Autodesk Inventor part; units mm, degrees
ref_plane "YZ Plane" through (0, 0, 0) normal (1, 0, 0) x (0, 1, 0)
ref_plane "XZ Plane" through (0, 0, 0) normal (0, 1, 0) x (-1, 0, 0)
ref_plane "XY Plane" through (0, 0, 0) normal (0, 0, 1) x (1, 0, 0)
sketch "Sketch1" plane through (0, 0, 0) normal (0, 1, 0) x (-1, 0, 0)
  line L0 (825, 12.5) -> (-825, 12.5)
  line L1 (-825, 12.5) -> (-825, -12.5)
  line L2 (-825, -12.5) -> (825, -12.5)
  line L3 (825, -12.5) -> (825, 12.5)
  line L4 (825, 12.5) -> (-825, -12.5) construction
  line L5 (-825, 12.5) -> (825, -12.5) construction
  point P0 (0, 0)
  dimension "d0" = 1650
  dimension "d1" = 25
extrude "Plate1" add sketch "Sketch1" along normal blind 3.2
sketch "Sketch2" plane through (825, 0, 9.3) normal (0, 0, 1) x (1, 0, 0)
  line L0 (-1650, 0) -> (0, 0)
  line L1 (0, 0) -> (0, 25)
  line L2 (0, 25) -> (-1650, 25)
  line L3 (-1650, 25) -> (-1650, 0)
edge flange "Flange1" height 25 angle 90 thickness 3.2 bend radius 1.516 thickness toward (0, 0, 1) relief tear relief width 3.2 relief depth 1.6 edges at (0, 3.2, 12.5) wall of the first edge with corners at (-825, 0, 9.3) (825, 0, 9.3) (825, 25, 9.3) (-825, 25, 9.3)
bend "Bend1"
corner "Corner1"
sketch "Sketch3" plane through (825, 25, 9.3) normal (0, 0, -1) x (-1, 0, 0)
  circle A0 centre (105, -10.45) radius 1.5706
  circle A1 centre (285, -10.45) radius 1.5706
  circle A2 centre (465, -10.45) radius 1.5706
  circle A3 centre (825, -10.45) radius 1.5706
  circle A4 centre (1005, -10.45) radius 1.5706
  circle A5 centre (1185, -10.45) radius 1.5706
  circle A6 centre (1365, -10.45) radius 1.5706
  circle A7 centre (1545, -10.45) radius 1.5706
  point P0 (825, -25)
hole "Hole1" at (540, 14.55, 9.3) at (720, 14.55, 9.3) at (360, 14.55, 9.3) at (0, 14.55, 9.3) at (-180, 14.55, 9.3) at (-360, 14.55, 9.3) at (-540, 14.55, 9.3) at (-720, 14.55, 9.3) direction (0, 0, 1) diameter 4.5 depth 3.2 tip angle 118
sketch "Sketch8" plane through (0, 0, 0) normal (0, -1, 0) x (1, 0, 0)
  line L0 (-825, -12.5) -> (825, -12.5)
  line L1 (0, -12.5) -> (0, -2.5)
  line L2 (0, -2.5) -> (-270, -2.5)
  line L3 (-270, -2.5) -> (-790, -2.5)
  line L4 (0, -2.5) -> (270, -2.5)
  line L5 (270, -2.5) -> (790, -2.5)
  point P0 (0, 0)
  dimension "d40" = 10
  dimension "d41" = 270
  dimension "d42" = 520
  dimension "d43" = 180
hole "Hole2" at (-790, 0, -2.5) at (-270, 0, -2.5) at (270, 0, -2.5) at (790, 0, -2.5) direction (0, 1, 0) diameter 4.5 depth 3.2 tip angle 118
fillet "Corner Round1" radius 3 4 edges at (825, 1.6, -12.5) (-825, 25, 10.9) (825, 25, 10.9) (-825, 1.6, -12.5)
sketch "Sketch9" plane through (825, 4.716, 9.3) normal (0, 0, -1) x (-1, 0, 0)
  circle A0 centre (644.759, 8.543) radius 2.5
  circle A1 centre (644.759, 8.543) radius 5.5
  point P0 (825, -4.716)
  dimension "d45" = 11
extrude "Cut3" cut sketch "Sketch9" against normal blind 3.2 contours A0 | A1
equation "\"d18\" = Thickness"
equation "\"d37\" = Thickness"
equation "\"d46\" = Thickness"
equation "\"d2\" = Thickness"
equation "\"d3\" = BendReliefWidth"
equation "\"d4\" = BendReliefDepth"
equation "\"d5\" = MinimumRemnant"
equation "\"d6\" = TransitionRadius"
equation "\"d9\" = BendRadius"
equation "\"d10\" = CornerReliefSize"
equation "\"d11\" = GapSize"
equation "\"d12\" = JacobiRadiusSize"
equation "\"BendReliefWidth\" = Thickness"
equation "\"BendReliefDepth\" = 0.5 * Thickness"
equation "\"CornerReliefSize\" = 4 * Thickness"
equation "\"MinimumRemnant\" = 2 * Thickness"
equation "\"TransitionRadius\" = BendRadius"
equation "\"JacobiRadiusSize\" = BendRadius"
equation "\"GapSize\" = Thickness"
properties part number "SP47V1 Chapa Acrilico Pasador"
Read the model definition and answer for the solid it produces. Units are mm, in the model's axes. Round coordinates to 2 decimals unless told otherwise and drop trailing zeros. Write each loop counter-clockwise with the first axis right and the second up, starting at its lowest first coordinate (ties: lowest second). Pieces come first, ordered by that corner, then holes.
1. The part is cut by section A-A, the plane x = -226.5. Determine the outline of the cut face in (y, z).
2. Given pin 1 Ø1 at (y, z) = (6.5, 9) entering from -X; pin 2 Ø2.5 at (x, z) = (-790, -2.5) entering from -Y; pin 3 Ø6 at (x, y) = (-540, 14.55) entering from -Z; pin 4 Ø4 at (x, z) = (-235.5, 10) entering from -Y, each flat-ended and moving along its own axis, determine where each tip first touches the part or whether it passes through.
3. Straight lines are drawn through the part: L1, parallel to X at y = 2.45, z = -2.5; L2, parallel to Y at x = -307, z = 2; L3, parallel to Z at x = 538, y = 8. For each, find the intervals that lie inside material, in ascending order.
Values:
1. outline: (0, -12.5) - (3.2, -12.5) - (3.2, 7.78) arc R1.52 cw to (4.72, 9.3) - (25, 9.3) - (25, 12.5) - (4.72, 12.5) arc R4.72 ccw to (0, 7.78) - close
2. pin 1: stops at x = -825
2. pin 2: passes through
2. pin 3: stops at z = 9.3
2. pin 4: stops at y = 0
3. L1: x = -825 to -792.25, -787.75 to -272.25, -267.75 to 267.75, 272.25 to 787.75, 792.25 to 825
3. L2: y = 0 to 3.2
3. L3: z = 9.3 to 12.5
